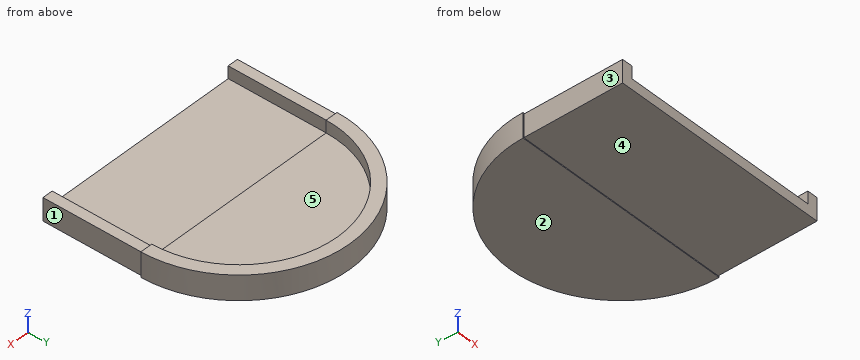
from build123d import *

# Parameters (mm, degrees)
F1_DEPTH = 3.175
F3_DEPTH = 3.175
F4_W     = 0.254
F4_H     = 25.4


with BuildPart() as f1:
    # F0 (on Top) → F1 (new body)
    with BuildSketch(Plane.XY):
        with BuildLine():
            Line((-3.175, 0), (0, 0))
            Line((0, 0), (0, 25.4))
            ThreePointArc((0, 25.4), (25.4, 50.8), (50.8, 25.4))
            Line((50.8, 25.4), (50.8, 0))
            Line((50.8, 0), (53.975, 0))
            Line((53.975, 0), (53.975, 25.4))
            ThreePointArc((53.975, 25.4), (25.4, 53.975), (-3.175, 25.4))
            Line((-3.175, 25.4), (-3.175, 0))
        make_face()
    extrude(amount=F1_DEPTH)

    # F2 (on face) → F3 (join)
    with BuildSketch(Plane(origin=(0, 0, 0), x_dir=(1, 0, 0), z_dir=(0, 0, -1))):
        with BuildLine():
            Line((53.975, -25.4), (53.975, 0))
            Line((53.975, 0), (-3.175, 0))
            Line((-3.175, 0), (-3.175, -25.4))
            ThreePointArc((-3.175, -25.4), (25.4, -53.975), (53.975, -25.4))
        make_face()
    extrude(amount=F3_DEPTH)

    # F5: sweep along a path in F5_path
    with BuildLine(Plane(origin=(-3.175, 0, 3.175), x_dir=(0, 0, -1), z_dir=(0, 1, 0))) as f5_path:
        Line((0, 0), (6.35, 0))
        Line((6.35, 0), (6.35, -57.15))
        Line((6.35, -57.15), (0, -57.15))
        Line((0, -57.15), (0, -53.975))
        Line((0, -53.975), (3.175, -53.975))
        Line((3.175, -53.975), (3.175, -3.175))
        Line((3.175, -3.175), (0, -3.175))
        Line((0, -3.175), (0, 0))
    # F4 (on face) → F5 (sweep, cut)
    with BuildSketch(Plane.XY.offset(3.175)):
        with Locations((-3.048, 12.7)):
            Rectangle(F4_W, F4_H)
    sweep(path=f5_path.line, transition=Transition.RIGHT, mode=Mode.SUBTRACT)


solid = f1.part
CAD build for the part. Positions are in the model's coordinates, mm. Face numbers are marked on the shaded views. A direction names the side the tool comes from. Give positions to 0.01 mm unless a question says otherwise; leave off trailing zeros. Write each loop counter-clockwise with the first axis right and the second up, starting at its lowest first coordinate (ties: lowest second). Pieces come first, ordered by that corner, then holes. Notation, with made-up numbers: M 75.5,14 L 84.5,14 A24 ccw 84.5,37 Z; hole C 9.25,39 d2. An arc over 180 degrees is marked long. Put each result on its own line as item: value. Start each with the question number.
(1) Flat gauge pins, fed straight in: pin 1 Ø3 at (y, z) = (11.5, 1.5) entering from +X; pin 2 Ø3 at (x, y) = (-2, 18.5) entering from +Z; pin 3 Ø5 at (x, y) = (23.5, 24.5) entering from +Z. Where does each tip first touch, or does it go through?
(2) Probe L1, parallel to X at y = 12.5, z = 2.75; L2, parallel to Z at x = 48, y = 22.5; L3, parallel to X at y = 34, z = 1.75. List the from-to ranges inside material, lowest first.
(3) Band-saw the part on D-D, the plane y = 50. Write the cut outline in (x, z) (3 decimals).
(4) Band-saw the part on C-C, the plane y = 19. Write the cut outline in (x, z), and give its area (3 significant figures).
(5) Which spindle directions (+Z, -Z, +X, -X, +Y, -Y) get a long thin tool onto all of the face, cutting with end or side? Do the marked faces 1, 2, 3, 4 and 5. Say none if no direction does.
(6) Band-saw the part on A-A, the plane z = 1. Write the cut outline in (x, y) (3 decimals), and give its area (3 significant figures).
(7) Band-saw the part on B-B, the plane x = 25.4. Write the cut outline in (y, z) (3 decimals), and give its area (3 significant figures).
Response values:
1. pin 1: stops at x = 53.72
1. pin 2: stops at z = 2.92
1. pin 3: stops at z = 0
2. L1: x = -2.92 to -0.25, 51.05 to 53.72
2. L2: z = -2.92 to -0.25
2. L3: x = -1.85 to 1.5, 49.3 to 52.65
3. outline: M 10.861,-3.175 L 39.939,-3.175 L 39.939,3.175 L 31.725,3.175 L 31.725,0 L 19.075,0 L 19.075,3.175 L 10.861,3.175 Z
4. outline: M -2.92,-2.92 L 53.72,-2.92 L 53.72,2.92 L 51.05,2.92 L 51.05,-0.25 L -0.25,-0.25 L -0.25,2.92 L -2.92,2.92 Z
4. area: 168 mm2
5. face 1: +Z, -Z, +X, -Y
5. face 2: -Z, +X, -X, +Y, -Y
5. face 3: +Z, -Z, -X, -Y
5. face 4: -Z, +X, -X, -Y
5. face 5: +Z, -Y
6. outline: M -3.175,25.4 L -2.921,25.4 L -2.921,0 L -0.254,0 L -0.254,25.4 L 0,25.4 A25.4 cw 50.8,25.4 L 51.054,25.4 L 51.054,0 L 53.721,0 L 53.721,25.4 L 53.975,25.4 A28.575 ccw Z
6. area: 405 mm2
7. outline: M 0,-2.921 L 25.4,-2.921 L 25.4,-3.175 L 53.975,-3.175 L 53.975,3.175 L 50.8,3.175 L 50.8,0 L 25.4,0 L 25.4,-0.254 L 0,-0.254 Z
7. area: 169 mm2
